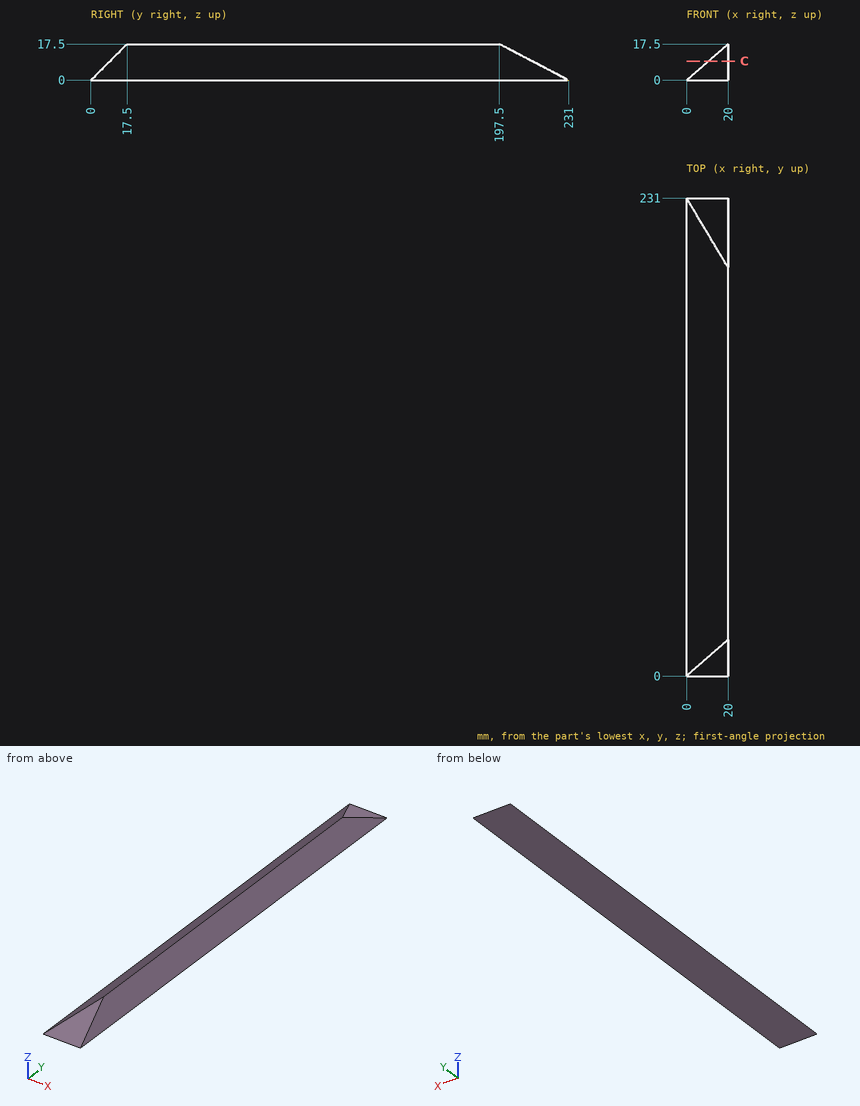
Could you check a few things on this drawing? It's one solid part, dimensions in mm from its lowest x, y, z. Coordinates: 2 decimals unless noted, no trailing zeros. Order: outer loops, then holes, each group sorted by start corner. A loop starts at its lowest first (then second) coordinate and runs counter-clockwise, first axis right, second up. Notation, with made-up numbers: M 60.25,67.5 L 115.25,67.5 A9 ccw 115.25,83.5 Z; hole C 19.5,-8 d10. An arc over 180 degrees is marked long. Answer as a JSON object with one key per item and string values. Group by question number.
(1) Suppose I cut it at C-C, the plane z = 9.25. Please give me the cut outline in (x, y).
(2) I need wall thicknesses on probe 1 along X at (y, z) = (213.5, 8); probe 2 along X at (y, z) = (85, 7); probe 3 along Y at (x, z) = (12.25, 5.75). Which ranges of each line are inside material? Lowest first, please.
(3) For pin 1 (8 mm diameter, centred on x = 14, y = 185.5, fed in from +Z); pin 2 (3 mm diameter, centred on x = 13, z = 5, fed in from -Y); pin 3 (5 mm diameter, centred on x = 7.5, y = 52, fed in from +Z), each with a flat end and sliding along its axis, tell me the tip position at first contact or that it passes through.
Values found:
{
 "1": {"outline": "M 10.57,9.25 L 20,9.25 L 20,213.29 L 10.57,213.29 Z"},
 "2": {"probe 1": "x = 9.14 to 20", "probe 2": "x = 8 to 20", "probe 3": "y = 5.75 to 219.99"},
 "3": {"pin 1": "stops at z = 15.75", "pin 2": "stops at y = 3.5", "pin 3": "stops at z = 8.75"}
}
